```python
from build123d import *

# Parameters (mm, degrees)
CHAMFER_1_SIZE      = 0.3
SKETCH_2_OUTSIDE_W  = 20.194
SKETCH_2_OUTSIDE_H  = 20.194
CUT_EXTRUDE_1_DEPTH = 14.709764028


with BuildPart() as part:
    # Sketch 1 → Revolve 1 (revolve)
    with BuildSketch(Plane.XY, mode=Mode.PRIVATE) as revolve_1_sk:
        Polygon((2.5, 0), (4, 0), (4, -4.5), (3.25, -4.5), (3.25, -6), (5.75, -6), (5.75, -10), (6.631652498, -10), (0.631652498, -16), (0.5, -15), (2.5, -12.616492815), align=None)
    revolve(revolve_1_sk.sketch.rotate(Axis((0, 8.266911596, 0), (0, -1, 0)), 90), axis=Axis((0, 8.266911596, 0), (0, -1, 0)))

    # Chamfer 1
    chamfer_1_edges = [part.edges().sort_by_distance(p)[0] for p in [
        (0, -10, -5.75),
        (0, -6, -5.75),
        (0, -4.5, -4),
        (0, 0, -4),
        (0, 0, -2.5),
    ]]
    chamfer(chamfer_1_edges, length=CHAMFER_1_SIZE)

    # Sketch 2 outside → Cut-Extrude 1 (cut, through all)
    with BuildSketch(Plane(origin=(0, -6, 0), x_dir=(1, 0, 0), z_dir=(0, 1, 0))):
        Rectangle(SKETCH_2_OUTSIDE_W, SKETCH_2_OUTSIDE_H)
        Polygon((5.773502692, 0), (2.886751346, 5), (-2.886751346, 5), (-5.773502692, 0), (-2.886751346, -5), (2.886751346, -5), align=None, mode=Mode.SUBTRACT)
    extrude(amount=-CUT_EXTRUDE_1_DEPTH, mode=Mode.SUBTRACT)


solid = part.part
```
Source: CAD feature listing. Evaluate the final solid. Frame: model axes, mm. A direction names the side the tool comes from. Coordinates: 2 decimals unless noted, no trailing zeros. Write each loop counter-clockwise with the first axis right and the second up, starting at its lowest first coordinate (ties: lowest second). Pieces come first, ordered by that corner, then holes. Notation, with made-up numbers: (62.5, 3) -> (111.5, 3) arc R12 ccw to (111.5, 21) -> close; hole circle Ø6 at (25.25, 6). An arc over 180 degrees is marked (long way). Return JSON: item names as keys, results as strings. Group by question number.
1) Ray query, line 1 along X through (y, z) = (-6.75, 0); line 2 along Y through (x, z) = (-3.25, 1); line 3 along X through (y, z) = (-8.25, 0.75). Return the intervals inside material, ascending.
2) Mould query, pull axis Z, two halves, no side actions, for faces 3 (the face through (4.35, -8.776, -2.465)), 4 (the face through (3.905, -2.277, -0.867)), 5 (the face through (-0.1, -6.4, -2.5)). Classes: +Z half, -Z half, draft (parallel to the pull), parting line (faces both ways), or undercut.
3) Section query A-A, the plane y = -9.5. Return loops of the section in (x, z), plus the area to 3 significant figures.
4) Set-up query: faces 1 (the face through (0.537, -15.382, -0.119)), 2 (the face through (-0.1, -6, 3.4)). Return all of +Z, -Z, +X, -X, +Y, -Y with unobstructed straight access to the full face (end or side cutting, diameter ignored); none if empty.
5) Section query B-B, the plane y = -3.25. Return loops of the section in (x, z), plus the area to 3 significant figures.
6) Contact query for flat-ended pins moving along their axis: P1, Ø1.5, axis at x = -3, y = -3.5, coming from the +Z side; P2, Ø1, axis at x = 3, z = -4, coming from the -Y side; P3, Ø3, axis at y = -9.5, z = 3, coming from the +X side. Output: stop coordinate, or through.
7) Section query C-C, the plane y = -13.25. Return loops of the section in (x, z), plus the area to 3 significant figures.
From the geometry:
{
 "1": {"line 1": "-5.75 to -2.5, 2.5 to 5.75", "line 2": "-13.23 to -6, -4.5 to 0", "line 3": "-5.34 to -2.38, 2.38 to 5.34"},
 "2": {"face 3": "-Z half", "face 4": "parting line", "face 5": "undercut"},
 "3": {"outline": "(-5.75, -0.04) -> (-2.91, -4.96) arc R5.75 ccw to (-2.84, -5) -> (2.84, -5) arc R5.75 ccw to (2.91, -4.96) -> (5.75, -0.04) arc R5.75 ccw to (5.75, 0.04) -> (2.91, 4.96) arc R5.75 ccw to (2.84, 5) -> (-2.84, 5) arc R5.75 ccw to (-2.91, 4.96) -> (-5.75, 0.04) arc R5.75 ccw to start; hole circle Ø5 at (0, 0)", "area": "67.0 mm²"},
 "4": {"face 1": "-Y", "face 2": "none"},
 "5": {"outline": "circle Ø8 at (0, 0); hole circle Ø5 at (0, 0)", "area": "30.6 mm²"},
 "6": {"P1": "z = 3.31", "P2": "y = -12.13", "P3": "x = 4.91"},
 "7": {"outline": "circle Ø6.76 at (0, 0); hole circle Ø3.94 at (0, 0)", "area": "23.8 mm²"}
}
